For this review, take the finished solid that the model builds, in its own axes (mm). Coordinates: 2 decimals unless noted, no trailing zeros. Write each loop counter-clockwise with the first axis right and the second up, starting at its lowest first coordinate (ties: lowest second). Pieces come first, ordered by that corner, then holes.
1) We need section C-C on z = 722. Write out the cut boundary in (x, y), then the cut area to 3 significant figures.
2) To check wall thickness, follow line 1 along Y through (x, z) = (7.5, 316); line 2 along Y through (x, z) = (-10.25, 155.5). State the ranges of each line that lie inside material, in increasing order.
3) Insertion check: P1, Ø4, axis at y = -10, z = 505, coming from the +X side; P2, Ø2, axis at x = 10, y = -1, coming from the -Z side. Each pin has a flat end and moves straight along its axis. Give the tip position at first contact, or say it passes through.
4) We need section A-A on x = 3. Write out the cut boundary in (y, z), then the cut area to 3 significant figures.
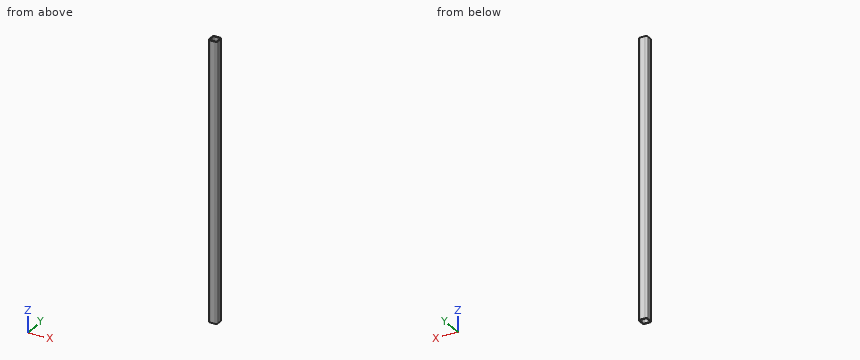
Autodesk Inventor part; units mm, degrees
ref_plane "Start Plane" through (0, 0, 15) normal (0, 0, 1) x (1, 0, 0)
ref_plane "End Plane" through (0, 0, 985) normal (0, 0, 1) x (1, 0, 0)
ref_plane "Work Plane4" through (-9, -2487, 15) normal (0, 0, -1) x (-1, 0, 0)
ref_plane "Start Plane" through (0, 0, 15) normal (0, 0, 1) x (1, 0, 0)
ref_plane "End Plane" through (0, 0, 985) normal (0, 0, 1) x (1, 0, 0)
sketch "Sketch" plane through (0, 0, 0) normal (0, 0, 1) x (1, 0, 0)
  line L0 (-15, -9) -> (-15, 9)
  line L1 (-9, 15) -> (9, 15)
  line L2 (15, 9) -> (15, -9)
  line L3 (9, -15) -> (-9, -15)
  arc A0 (-15, -9) -> (-9, -15) centre (-9, -9) ccw
  arc A1 (-9, 15) -> (-15, 9) centre (-9, 9) ccw
  arc A2 (15, 9) -> (9, 15) centre (9, 9) ccw
  arc A3 (9, -15) -> (15, -9) centre (9, -9) ccw
  arc A4 (-9, 12) -> (-12, 9) centre (-9, 9) ccw
  line L4 (-9, 12) -> (9, 12)
  arc A5 (12, 9) -> (9, 12) centre (9, 9) ccw
  line L5 (12, 9) -> (12, -9)
  arc A6 (9, -12) -> (12, -9) centre (9, -9) ccw
  line L6 (9, -12) -> (-9, -12)
  arc A7 (-12, -9) -> (-9, -12) centre (-9, -9) ccw
  line L7 (-12, -9) -> (-12, 9)
  line L8 (0, 22.7397) -> (0, -22.7397) construction
  line L9 (-22.7397, 0) -> (22.7397, 0) construction
  dimension "d7" = 6
  dimension "d10" = 30
  dimension "d11" = 30
  dimension "d12" = 3
  dimension "d15" = 15
  dimension "d16" = 15
extrude "Body" add sketch "Sketch" along normal up to surface (970 mm away) from surface at 15
sketch "Sketch3" plane through (0, 0, 0) normal (0, 0, 1) x (1, 0, 0)
  line L0 (0, 0) -> (10, 0)
ref_plane "Work Plane3" through (0, 0, 0) normal (0, -1, 0) x (1, 0, 0)
ref_plane "Work Plane4" through (-9, -2487, 15) normal (0, 0, -1) x (-1, 0, 0)
split "Split1" plane through (-9, -2487, 15) removes the side toward (0, 0, -1)
ref_plane "Work Plane5" through (9, -2487, 985) normal (0, 0, 1) x (1, 0, 0)
split "Split2" plane through (9, -2487, 985) removes the side toward (0, 0, 1)
sketch "Sketch4" plane through (0, 0, 0) normal (0, -1, 0) x (1, 0, 0)
  line L0 (-2, 15) -> (12, 15)
  line L1 (-2, 985) -> (12, 985)
  dimension "d18" = 970
equation "\"d7\" = G_IR"
equation "\"d10\" = G_H"
equation "\"d11\" = G_W"
equation "\"d12\" = G_T"
equation "\"d15\" = 0.5 * d10"
equation "\"d16\" = 0.5 * d11"
equation "\"d3\" = G_L"
equation "\"G_W\" = 30"
equation "\"G_H\" = 30"
equation "\"G_T\" = 3"
equation "\"G_IR\" = 6"
equation "\"G_L\" = d18"
equation "\"G_OFFSET_START\" = -15"
equation "\"G_OFFSET_END\" = -15"
equation "\"d13\" = -G_OFFSET_START"
equation "\"d14\" = G_OFFSET_END + B_L"
properties part number "DIN EN 10219-2 - 30 x 30 x 3  - 970" material "Steel, Mild"
Result:
1. outline: (-15, -9) arc R6 ccw to (-9, -15) - (9, -15) arc R6 ccw to (15, -9) - (15, 9) arc R6 ccw to (9, 15) - (-9, 15) arc R6 ccw to (-15, 9) - close; hole (-12, -9) arc R3 ccw to (-9, -12) - (9, -12) arc R3 ccw to (12, -9) - (12, 9) arc R3 ccw to (9, 12) - (-9, 12) arc R3 ccw to (-12, 9) - close
1. area: 301 mm2
2. line 1: y = -15 to -12, 12 to 15
2. line 2: y = -14.87 to -11.73, 11.73 to 14.87
3. P1: stops at x = 15
3. P2: passes through
4. outline: (-15, 15) - (-12, 15) - (-12, 985) - (-15, 985) - close; (12, 15) - (15, 15) - (15, 985) - (12, 985) - close
4. area: 5,820 mm2
